Here's how the part is built. I have some questions about the finished solid (model axes, mm). Round coordinates to 2 decimals unless told otherwise and drop trailing zeros. Order: outer loops, then holes, each group sorted by start corner. A loop starts at its lowest first (then second) coordinate and runs counter-clockwise, first axis right, second up. Notation, with made-up numbers: (47.5, 6.25) - (101.5, 6.25) arc R20 cw to (101.5, 40.25) - close; hole circle Ø3 at (45.5, 72). An arc over 180 degrees is marked (long way). One line per item, written item: value.
from build123d import *

# Parameters (mm, degrees)
BOSS_EXTRUDE1_DEPTH     = 0.8
ADDTOLERANCE_DEPTH      = 71.715203457
ADDTOLERANCE_DEPTH_BACK = 71.715203457
CUT_EXTRUDE1_DEPTH      = 71.573791169
CUT_EXTRUDE1_DEPTH_BACK = 71.573791169


with BuildPart() as part:
    # Sketch2 → Boss-Extrude1 (new, symmetric)
    with BuildSketch(Plane(origin=(0, 0, 0), x_dir=(1, 0, 0), z_dir=(0, 1, 0))):
        Polygon((41.5, -47.4), (47.4, -41.5), (50, -41.5), (50, 41.5), (47.4, 41.5), (47.4, 46.4), (37, 46.4), (37, 50), (-37, 50), (-37, 46.4), (-47.4, 46.4), (-47.4, 41.5), (-50, 41.5), (-50, -41.5), (-47.4, -41.5), (-41.5, -47.4), align=None)
    extrude(amount=BOSS_EXTRUDE1_DEPTH, both=True)

    # Sketch3 → AddTolerance (cut, two sides: drawn at the far end of the back side and taken through both)
    with BuildSketch(Plane(origin=(0, 0, 0), x_dir=(1, 0, 0), z_dir=(0, 1, 0)).offset(-ADDTOLERANCE_DEPTH_BACK)):
        Polygon((37, 50), (-37, 50), (-37, 46.4), (-47.4, 46.4), (-47.4, 41.5), (-50, 41.5), (-50, -41.5), (-47.4, -41.5), (-47.5, -41.4), (-49.9, -41.4), (-49.9, 41.4), (-47.3, 41.4), (-47.3, 46.3), (-36.9, 46.3), (-36.9, 49.9), (36.9, 49.9), (36.9, 46.3), (47.3, 46.3), (47.3, 41.4), (49.9, 41.4), (49.9, -41.4), (47.5, -41.4), (47.4, -41.5), (50, -41.5), (50, 41.5), (47.4, 41.5), (47.4, 46.4), (37, 46.4), align=None)
    extrude(amount=ADDTOLERANCE_DEPTH + ADDTOLERANCE_DEPTH_BACK, mode=Mode.SUBTRACT)

    # Sketch4 → Cut-Extrude1 (cut, two sides: drawn at the far end of the back side and taken through both)
    with BuildSketch(Plane(origin=(0, 0, 0), x_dir=(1, 0, 0), z_dir=(0, 1, 0)).offset(-CUT_EXTRUDE1_DEPTH_BACK)):
        Polygon((-41.5, -47.4), (41.5, -47.4), (43.1, -45.8), (-43.1, -45.8), align=None)
        Polygon((-43.1, -45.8), (43.1, -45.8), (44.1, -44.8), (-44.1, -44.8), align=None)
    extrude(amount=CUT_EXTRUDE1_DEPTH + CUT_EXTRUDE1_DEPTH_BACK, mode=Mode.SUBTRACT)


solid = part.part
Q1. If I drill on line 1 along Z through (x, y) = (41.5, 0.3), over which ranges is the centre line in solid material (lowest first)?
Results list:
line 1: -46.3 to 44.8
Q2. If we section it at A-A, the plane y = 0: Please give me the cut outline in (x, z).
Results list:
outline: (-49.9, -41.4) - (-47.3, -41.4) - (-47.3, -46.3) - (-36.9, -46.3) - (-36.9, -49.9) - (36.9, -49.9) - (36.9, -46.3) - (47.3, -46.3) - (47.3, -41.4) - (49.9, -41.4) - (49.9, 41.4) - (47.5, 41.4) - (44.1, 44.8) - (-44.1, 44.8) - (-47.5, 41.4) - (-49.9, 41.4) - close
Q3. If we section it at B-B, the plane z = -43: Please give me the cut outline in (x, y).
Results list:
outline: (-47.3, -0.8) - (47.3, -0.8) - (47.3, 0.8) - (-47.3, 0.8) - close
Q4. Will these pins go through, and if not, where does the flat tip stop? pin 1 (0.8 mm diameter, centred on y = 0, z = -44, fed in from +X); pin 2 (0.8 mm diameter, centred on x = 48.5, y = 0, fed in from +Z); pin 3 (0.8 mm diameter, centred on y = -0.5, z = -47.5, fed in from -X).
Results list:
pin 1: x = 47.3
pin 2: z = 41.4
pin 3: x = -36.9
